```python
from build123d import *

# Parameters (mm, degrees)
SKETCH1_W                     = 17.8
SKETCH1_H                     = 15.8
BOSS_EXTRUDE1_DEPTH           = 1.5
SKETCH2_W                     = 7.103176806
SKETCH2_H                     = 5.754981775
BOSS_EXTRUDE2_DEPTH           = 1
SKETCH3_R                     = 0.75
BOSS_EXTRUDE3_DEPTH           = 0.8
BOSS_EXTRUDE3_DRAFT           = 20
BOSS_EXTRUDE3_PROFILE_2_DEPTH = 0.8
BOSS_EXTRUDE3_PROFILE_2_DRAFT = 20
BOSS_EXTRUDE3_PROFILE_3_DEPTH = 0.8
BOSS_EXTRUDE3_PROFILE_3_DRAFT = 20
BOSS_EXTRUDE3_PROFILE_4_DEPTH = 0.8
BOSS_EXTRUDE3_PROFILE_4_DRAFT = 20
BOSS_EXTRUDE3_PROFILE_5_DEPTH = 0.8
BOSS_EXTRUDE3_PROFILE_5_DRAFT = 20
BOSS_EXTRUDE3_PROFILE_6_DEPTH = 0.8
BOSS_EXTRUDE3_PROFILE_6_DRAFT = 20


with BuildPart() as part:
    # Sketch1 → Boss-Extrude1 (new body)
    with BuildSketch(Plane(origin=(0, 0, 0), x_dir=(1, 0, 0), z_dir=(0, 1, 0))):
        Rectangle(SKETCH1_W, SKETCH1_H)
    extrude(amount=BOSS_EXTRUDE1_DEPTH)

    # Sketch2 → Boss-Extrude2 (add)
    with BuildSketch(Plane(origin=(0, 1.5, 0), x_dir=(1, 0, 0), z_dir=(0, 1, 0))):
        with Locations((-1.036299166, 0.010061156)):
            Rectangle(SKETCH2_W, SKETCH2_H)
    extrude(amount=BOSS_EXTRUDE2_DEPTH)


with BuildPart() as boss_extrude3_tool:
    # Sketch3 → Boss-Extrude3 (with draft: the straight prism first)
    with BuildSketch(Plane(origin=(0, 1.5, 0), x_dir=(1, 0, 0), z_dir=(0, 1, 0))):
        with Locations((7.12329912, 6.4)):
            Circle(SKETCH3_R)
    extrude(amount=BOSS_EXTRUDE3_DEPTH)
    # Boss-Extrude3: the draft: its side faces are tilted about the plane it starts from
    boss_extrude3_sides = [boss_extrude3_tool.faces().sort_by_distance(p)[0] for p in [
        (6.37329912, 1.9, -6.4),
    ]]
    draft(boss_extrude3_sides, Plane(origin=(0, 1.5, 0), x_dir=(1, 0, 0), z_dir=(0, 1, 0)), BOSS_EXTRUDE3_DRAFT)


with BuildPart() as part_1:
    add(part.part)

    # Boss-Extrude3: add boss_extrude3_tool
    add(boss_extrude3_tool.part)


with BuildPart() as boss_extrude3_profile_2_tool:
    # Sketch3 → Boss-Extrude3 profile 2 (with draft: the straight prism first)
    with BuildSketch(Plane(origin=(0, 1.5, 0), x_dir=(1, 0, 0), z_dir=(0, 1, 0))):
        with Locations((7.12329912, 3.9)):
            Circle(SKETCH3_R)
    extrude(amount=BOSS_EXTRUDE3_PROFILE_2_DEPTH)
    # Boss-Extrude3 profile 2: the draft: its side faces are tilted about the plane it starts from
    boss_extrude3_profile_2_sides = [boss_extrude3_profile_2_tool.faces().sort_by_distance(p)[0] for p in [
        (6.37329912, 1.9, -3.9),
    ]]
    draft(boss_extrude3_profile_2_sides, Plane(origin=(0, 1.5, 0), x_dir=(1, 0, 0), z_dir=(0, 1, 0)), BOSS_EXTRUDE3_PROFILE_2_DRAFT)


with BuildPart() as part_2:
    add(part_1.part)

    # Boss-Extrude3 profile 2: add boss_extrude3_profile_2_tool
    add(boss_extrude3_profile_2_tool.part)


with BuildPart() as boss_extrude3_profile_3_tool:
    # Sketch3 → Boss-Extrude3 profile 3 (with draft: the straight prism first)
    with BuildSketch(Plane(origin=(0, 1.5, 0), x_dir=(1, 0, 0), z_dir=(0, 1, 0))):
        with Locations((7.12329912, 1.4)):
            Circle(SKETCH3_R)
    extrude(amount=BOSS_EXTRUDE3_PROFILE_3_DEPTH)
    # Boss-Extrude3 profile 3: the draft: its side faces are tilted about the plane it starts from
    boss_extrude3_profile_3_sides = [boss_extrude3_profile_3_tool.faces().sort_by_distance(p)[0] for p in [
        (6.37329912, 1.9, -1.4),
    ]]
    draft(boss_extrude3_profile_3_sides, Plane(origin=(0, 1.5, 0), x_dir=(1, 0, 0), z_dir=(0, 1, 0)), BOSS_EXTRUDE3_PROFILE_3_DRAFT)


with BuildPart() as part_3:
    add(part_2.part)

    # Boss-Extrude3 profile 3: add boss_extrude3_profile_3_tool
    add(boss_extrude3_profile_3_tool.part)


with BuildPart() as boss_extrude3_profile_4_tool:
    # Sketch3 → Boss-Extrude3 profile 4 (with draft: the straight prism first)
    with BuildSketch(Plane(origin=(0, 1.5, 0), x_dir=(1, 0, 0), z_dir=(0, 1, 0))):
        with Locations((7.12329912, -1.1)):
            Circle(SKETCH3_R)
    extrude(amount=BOSS_EXTRUDE3_PROFILE_4_DEPTH)
    # Boss-Extrude3 profile 4: the draft: its side faces are tilted about the plane it starts from
    boss_extrude3_profile_4_sides = [boss_extrude3_profile_4_tool.faces().sort_by_distance(p)[0] for p in [
        (6.37329912, 1.9, 1.1),
    ]]
    draft(boss_extrude3_profile_4_sides, Plane(origin=(0, 1.5, 0), x_dir=(1, 0, 0), z_dir=(0, 1, 0)), BOSS_EXTRUDE3_PROFILE_4_DRAFT)


with BuildPart() as part_4:
    add(part_3.part)

    # Boss-Extrude3 profile 4: add boss_extrude3_profile_4_tool
    add(boss_extrude3_profile_4_tool.part)


with BuildPart() as boss_extrude3_profile_5_tool:
    # Sketch3 → Boss-Extrude3 profile 5 (with draft: the straight prism first)
    with BuildSketch(Plane(origin=(0, 1.5, 0), x_dir=(1, 0, 0), z_dir=(0, 1, 0))):
        with Locations((7.12329912, -3.6)):
            Circle(SKETCH3_R)
    extrude(amount=BOSS_EXTRUDE3_PROFILE_5_DEPTH)
    # Boss-Extrude3 profile 5: the draft: its side faces are tilted about the plane it starts from
    boss_extrude3_profile_5_sides = [boss_extrude3_profile_5_tool.faces().sort_by_distance(p)[0] for p in [
        (6.37329912, 1.9, 3.6),
    ]]
    draft(boss_extrude3_profile_5_sides, Plane(origin=(0, 1.5, 0), x_dir=(1, 0, 0), z_dir=(0, 1, 0)), BOSS_EXTRUDE3_PROFILE_5_DRAFT)


with BuildPart() as part_5:
    add(part_4.part)

    # Boss-Extrude3 profile 5: add boss_extrude3_profile_5_tool
    add(boss_extrude3_profile_5_tool.part)


with BuildPart() as boss_extrude3_profile_6_tool:
    # Sketch3 → Boss-Extrude3 profile 6 (with draft: the straight prism first)
    with BuildSketch(Plane(origin=(0, 1.5, 0), x_dir=(1, 0, 0), z_dir=(0, 1, 0))):
        with Locations((7.12329912, -6.1)):
            Circle(SKETCH3_R)
    extrude(amount=BOSS_EXTRUDE3_PROFILE_6_DEPTH)
    # Boss-Extrude3 profile 6: the draft: its side faces are tilted about the plane it starts from
    boss_extrude3_profile_6_sides = [boss_extrude3_profile_6_tool.faces().sort_by_distance(p)[0] for p in [
        (6.37329912, 1.9, 6.1),
    ]]
    draft(boss_extrude3_profile_6_sides, Plane(origin=(0, 1.5, 0), x_dir=(1, 0, 0), z_dir=(0, 1, 0)), BOSS_EXTRUDE3_PROFILE_6_DRAFT)


with BuildPart() as part_6:
    add(part_5.part)

    # Boss-Extrude3 profile 6: add boss_extrude3_profile_6_tool
    add(boss_extrude3_profile_6_tool.part)


solid = part_6.part
```
Can you work these out from the model? Positions are in its coordinate system, mm. A direction names the side the tool comes from. Round coordinates to 2 decimals unless told otherwise and drop trailing zeros. Loops run counter-clockwise (first coordinate to the right, second up) from the corner with the lowest first, then second, coordinate; pieces in that order, holes last.
Item 1: Suppose I cut it at C-C, the plane z = -6.4. Write out the boundary of the cut face in (x, y).
Item 2: Suppose I cut it at A-A, the plane z = 1.1. Write out the boundary of the cut face in (x, y).
Item 3: If we mould it in two halves opening along Z, with no side actions, what happens to faces 1 (the flat face through (7.1, 2.3, 3.6)), 2 (the flat face through (-1, 2, -2.888)), 3 (the conical face through (7.624, 2.072, 1.307))? For each: +Z half, -Z half, draft (parallel to the pull), parting line (faces both ways), or undercut.
Item 4: Suppose I cut it at D-D, the plane z = 5. Write out the boundary of the cut face in (x, y).
Item 5: Suppose I cut it at B-B, the plane x = -7.75. Write out the boundary of the cut face in (y, z), then the cut area to 3 significant figures.
Item 6: Will these pins go through, and if not, where does the flat tip stop? pin 1 Ø3 at (x, z) = (-6.5, 6) entering from +Y; pin 2 Ø0.7 at (x, z) = (7, 6) entering from +Y; pin 3 Ø0.5 at (x, y) = (0.5, 2) entering from +Z.
Item 7: Please list where these lines run through material, in increasing order: L1, parallel to Y at x = -7.25, z = -1; L2, parallel to X at y = 1.8, z = 2; L3, parallel to Y at x = 7.25, z = -1.
Item 8: Which directions (+Z, -Z, +X, -X, +Y, -Y) give clear straight access to the entire face, cutting with the end or side of a thin tool? Please do faces 4 (the flat face through (0, 0, 0)), 5 (the flat face through (2.515, 2, 0)), 6 (the flat face through (7.1, 2.3, -1.4)), 7 (the flat face through (0, 1.5, -4)).
Reported:
1. outline: (-8.9, 0) - (8.9, 0) - (8.9, 1.5) - (7.87, 1.5) - (7.58, 2.3) - (6.66, 2.3) - (6.37, 1.5) - (-8.9, 1.5) - close
2. outline: (-8.9, 0) - (8.9, 0) - (8.9, 1.5) - (7.87, 1.5) - (7.58, 2.3) - (6.66, 2.3) - (6.37, 1.5) - (2.52, 1.5) - (2.52, 2.5) - (-4.59, 2.5) - (-4.59, 1.5) - (-8.9, 1.5) - close
3. face 1: draft
3. face 2: -Z half
3. face 3: undercut
4. outline: (-8.9, 0) - (8.9, 0) - (8.9, 1.5) - (-8.9, 1.5) - close
5. outline: (0, -7.9) - (1.5, -7.9) - (1.5, 7.9) - (0, 7.9) - close
5. area: 23.7 mm2
6. pin 1: stops at y = 1.5
6. pin 2: stops at y = 2.3
6. pin 3: stops at z = 2.87
7. L1: y = 0 to 1.5
7. L2: x = -4.59 to 2.52
7. L3: y = 0 to 2.3
8. face 4: +Z, -Z, +X, -X, -Y
8. face 5: +Z, -Z, +Y
8. face 6: +Z, -Z, +X, +Y
8. face 7: +Y
